from build123d import *

# Parameters (mm, degrees)
SKETCH3_R           = 31.55
BOSS_EXTRUDE1_DEPTH = 13
SKETCH6_R           = 31.55
BOSS_EXTRUDE2_DEPTH = 54
FILLET1_R           = 2.54
SKETCH7_R           = 5
BOSS_EXTRUDE3_DEPTH = 30


with BuildPart() as part:
    # Sketch3 → Boss-Extrude1 (new body)
    with BuildSketch(Plane(origin=(0, 0, 0), x_dir=(1, 0, 0), z_dir=(0, 1, 0))):
        Circle(SKETCH3_R)
    extrude(amount=BOSS_EXTRUDE1_DEPTH)

    # Sketch5 → Cut-Revolve1 (revolve, cut)
    with BuildSketch(Plane.XY):
        Polygon((31.55, 13), (26.55, 13), (31.55, 0), align=None)
    revolve(axis=Axis((0, 13, 0), (0, -1, 0)), mode=Mode.SUBTRACT)

    # Sketch6 → Boss-Extrude2 (add)
    with BuildSketch(Plane.XZ):
        Circle(SKETCH6_R)
    extrude(amount=BOSS_EXTRUDE2_DEPTH)

    # Fillet1
    fillet1_edges = [part.edges().sort_by_distance(p)[0] for p in [
        (-31.55, -54, 0),
        (-26.55, 13, 0),
    ]]
    fillet(fillet1_edges, radius=FILLET1_R)

    # Sketch7 → Boss-Extrude3 (add)
    with BuildSketch(Plane(origin=(0, 13, 0), x_dir=(1, 0, 0), z_dir=(0, 1, 0))):
        Circle(SKETCH7_R)
    extrude(amount=BOSS_EXTRUDE3_DEPTH)


solid = part.part
Geometry check sheet. Reference: the model listing, model coordinates, mm. A direction names the side the tool comes from. Round coordinates to 2 decimals unless told otherwise and drop trailing zeros. Order: outer loops, then holes, each group sorted by start corner. A loop starts at its lowest first (then second) coordinate and runs counter-clockwise, first axis right, second up. Notation, with made-up numbers: M 64.5,-23.5 L 68.5,-23.5 A22 ccw 68.5,-0.5 Z; hole C 16,85.5 d3. An arc over 180 degrees is marked long. Write each question's results on one line, items separated by ' | '. Start each with the question number.
1. Go/stop test with flat-tipped pins: P1, Ø1.5, axis at y = 32.5, z = 2.5, coming from the -X side; P2, Ø1, axis at x = -6.5, y = -7.5, coming from the +Z side; P3, Ø1, axis at x = 1, y = -33.5, coming from the +Z side. Record where each tip stops, or that it passes through.
2. Set-up check for faces 1 (the face through (-1.08, 27.79, 4.88)), 2 (the face through (-25.037, -25.37, -19.198)): record each of +Z, -Z, +X, -X, +Y, -Y from which the full face is reachable in a straight line by a thin tool's end or side.
3. Cross-section at A-A on x = 0. Record the boundary of the cut face in (y, z), plus the area to 3 significant figures.
4. Material ranges on L1, parallel to Y at x = 20, z = 0.5; L2, parallel to X at y = -2, z = 19.5; L3, parallel to Y at x = -15.5, z = 25, recorded low to high. Write a range as from..to.
5. Cross-section at B-B on z = 0. Record the boundary of the cut face in (x, y).
6. Cross-section at D-D on y = 8. Record the boundary of the cut face in (x, z).
7. Cross-section at C-C on y = -7. Record the boundary of the cut face in (x, z), plus the area to 3 significant figures.
Resolved:
1) P1: x = -4.68 | P2: z = 30.97 | P3: z = 31.55
2) face 1: +Y | face 2: +Y, -Y
3) outline: M -54,-29.01 A2.54 ccw -51.46,-31.55 L 0,-31.55 L 11.37,-27.18 A2.54 ccw 13,-24.81 L 13,-5 L 43,-5 L 43,5 L 13,5 L 13,24.81 A2.54 ccw 11.37,27.18 L 0,31.55 L -51.46,31.55 A2.54 ccw -54,29.01 Z | area: 4,460 mm2
4) L1: -54..13 | L2: -24.8..24.8 | L3: -53.97..5.55
5) outline: M -31.55,-51.46 A2.54 ccw -29.01,-54 L 29.01,-54 A2.54 ccw 31.55,-51.46 L 31.55,0 L 27.18,11.37 A2.54 ccw 24.81,13 L 5,13 L 5,43 L -5,43 L -5,13 L -24.81,13 A2.54 ccw -27.18,11.37 L -31.55,0 Z
6) outline: C 0,0 d56.95
7) outline: C 0,0 d63.1 | area: 3,130 mm2
